Job drawing, mm, ordinate dimensions from the low corner. One solid piece. A direction names the side the tool comes from. Coordinates: 2 decimals unless noted, no trailing zeros. Write each loop counter-clockwise with the first axis right and the second up, starting at its lowest first coordinate (ties: lowest second). Pieces come first, ordered by that corner, then holes. Notation, with made-up numbers: (-21, 62) -> (-2, 62) arc R17 cw to (-2, 79) -> close; hole circle Ø2 at (81.25, 76). An arc over 180 degrees is marked (long way). Answer as a JSON object with one key per item and string values. Group by question number.
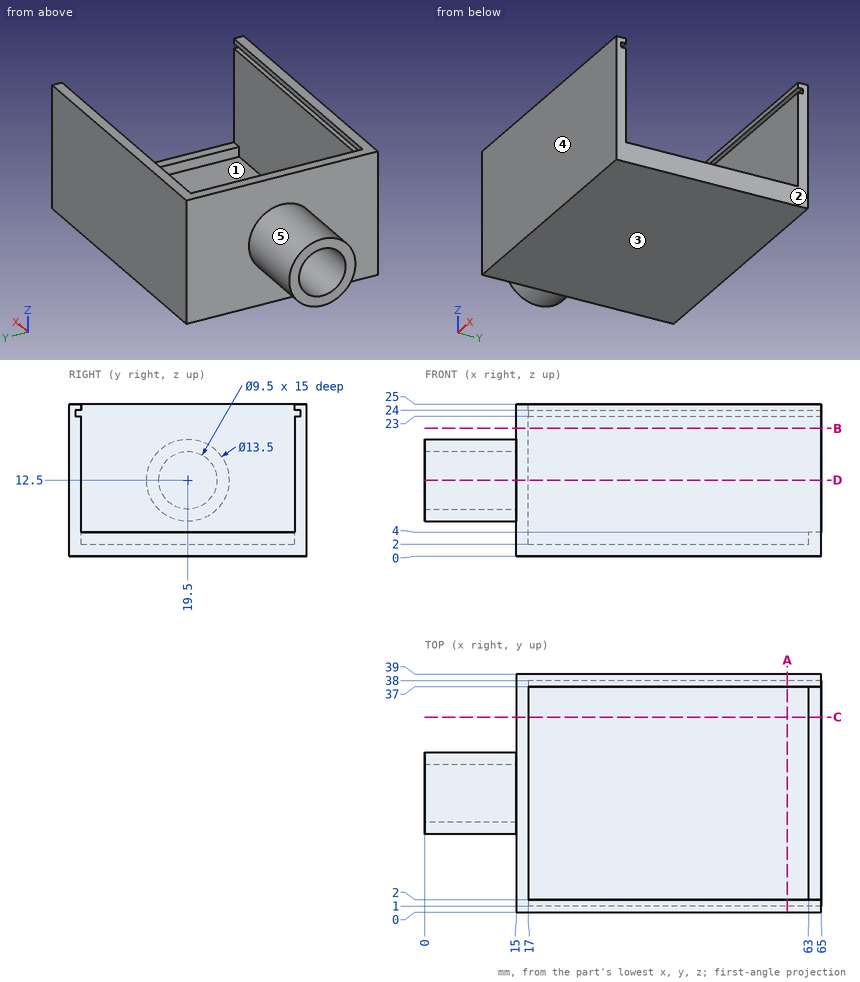
(1) Cut at D-D on z = 12.5. List the corners of the cut face in (x, y).
(2) Pull direction X, two halves, no side cores. Call the marked faces 1, 2 and 3: released by +X, released by -X, zero draft, split by the parting line, or undercut.
(3) 3-axis set-ups, long thin cutter, end or side, ignore diameter. For the marked faces 4 and 5: which of +Z, -Z, +X, -X, +Y, -Y reach the whole face in a straight line?
(4) Cut at C-C on y = 32. List the corners of the cut face in (x, z), plus the area to 3 significant figures.
(5) Cut at A-A on x = 59.5. List the corners of the cut face in (y, z), plus the area to 3 significant figures.
(6) Pin check, flat tips, straight feed: pin 1 (0.6 mm diameter, centred on y = 27.5, z = 2.5, fed in from -X); pin 2 (2 mm diameter, centred on x = 64.5, y = 16.5, fed in from +Z); pin 3 (10.5 mm diameter, centred on x = 31.5, y = 24.5, fed in from +Z). Stop position of each tip, or through.
(7) Cut at B-B on z = 21. List the corners of the cut face in (x, y).
(8) Wall check: probe 1 along X at (y, z) = (4.5, 2.75); probe 2 along Y at (x, z) = (30, 13.75); probe 3 along X at (y, z) = (6.5, 23). Give the ranges that are in metal, low to high.
Results found:
{
 "1": {"outline": "(0, 12.75) -> (15, 12.75) -> (15, 0) -> (65, 0) -> (65, 2) -> (17, 2) -> (17, 37) -> (65, 37) -> (65, 39) -> (15, 39) -> (15, 26.25) -> (0, 26.25) -> (0, 24.25) -> (15, 24.25) -> (15, 14.75) -> (0, 14.75) -> close"},
 "2": {"face 1": "undercut", "face 2": "released by +X", "face 3": "zero draft"},
 "3": {"face 4": "+Z, -Z, +X, -X, -Y", "face 5": "-X"},
 "4": {"outline": "(15, 0) -> (65, 0) -> (65, 4) -> (63, 4) -> (63, 2) -> (17, 2) -> (17, 25) -> (15, 25) -> close", "area": "150 mm²"},
 "5": {"outline": "(0, 0) -> (39, 0) -> (39, 25) -> (37, 25) -> (37, 24) -> (38, 24) -> (38, 23) -> (37, 23) -> (37, 2) -> (2, 2) -> (2, 23) -> (1, 23) -> (1, 24) -> (2, 24) -> (2, 25) -> (0, 25) -> close", "area": "168 mm²"},
 "6": {"pin 1": "stops at x = 15", "pin 2": "stops at z = 4", "pin 3": "stops at z = 2"},
 "7": {"outline": "(15, 0) -> (65, 0) -> (65, 2) -> (17, 2) -> (17, 37) -> (65, 37) -> (65, 39) -> (15, 39) -> close"},
 "8": {"probe 1": "x = 15 to 17, 63 to 65", "probe 2": "y = 0 to 2, 37 to 39", "probe 3": "x = 15 to 17"}
}
